from build123d import *

# Parameters (mm, degrees)
SKETCH1_R           = 1.73
BOSS_EXTRUDE1_DEPTH = 116
DOME1_FACE_RADIUS   = 1.73
DOME1_HEIGHT        = 5
DOME2_FACE_RADIUS   = 1.73
DOME2_HEIGHT        = 5


with BuildPart() as part:
    # Sketch1 → Boss-Extrude1 (new body)
    with BuildSketch(Plane.XY):
        with Locations(Location((0, 0, 0), (0, 0, 180))):
            Circle(SKETCH1_R)
    extrude(amount=BOSS_EXTRUDE1_DEPTH)

    # Dome1: a dome of height H over a round flat face of radius A is a cap of a sphere of radius (A * A + H * H) / (2 * H)
    dome1_r = (DOME1_FACE_RADIUS * DOME1_FACE_RADIUS + DOME1_HEIGHT * DOME1_HEIGHT) / (2 * DOME1_HEIGHT)
    dome1_base = Plane((0, 0, 0), z_dir=(0, 0, -1))
    with Locations(dome1_base.offset(DOME1_HEIGHT - dome1_r)):
        dome1_ball = Sphere(dome1_r, mode=Mode.PRIVATE)
    add(split(dome1_ball, bisect_by=dome1_base, keep=Keep.TOP, mode=Mode.PRIVATE))

    # Dome2: a dome of height H over a round flat face of radius A is a cap of a sphere of radius (A * A + H * H) / (2 * H)
    dome2_r = (DOME2_FACE_RADIUS * DOME2_FACE_RADIUS + DOME2_HEIGHT * DOME2_HEIGHT) / (2 * DOME2_HEIGHT)
    dome2_base = Plane((0, 0, 116), z_dir=(0, 0, 1))
    with Locations(dome2_base.offset(DOME2_HEIGHT - dome2_r)):
        dome2_ball = Sphere(dome2_r, mode=Mode.PRIVATE)
    add(split(dome2_ball, bisect_by=dome2_base, keep=Keep.TOP, mode=Mode.PRIVATE))


solid = part.part
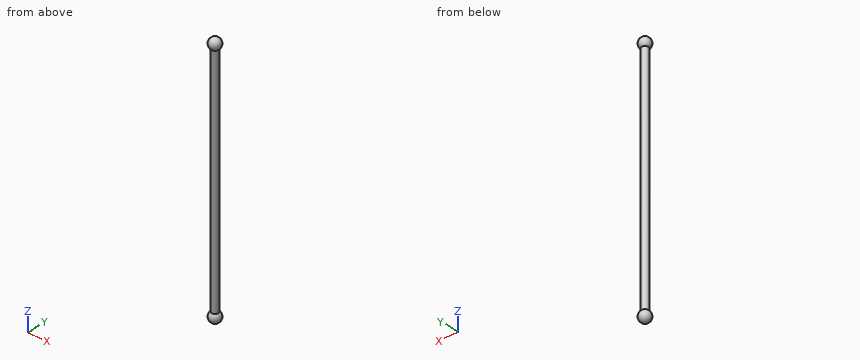
Input: part model. Units: mm. Frame: model coordinates. Round coordinates to 2 decimals unless told otherwise and drop trailing zeros. Loops run counter-clockwise (first coordinate to the right, second up) from the corner with the lowest first, then second, coordinate; pieces in that order, holes last. Notation, with made-up numbers: M 75.5,-23 L 83.5,-23 A9 cw 83.5,-7 Z; hole C 16,43 d8. An arc over 180 degrees is marked long. Answer as CSV lines item,"result". Start each with the question number.
(1) First-contact query: pin 1 (1.5 mm diameter, centred on x = 0, z = 54.5, fed in from +Y); pin 2 (1 mm diameter, centred on x = 0.5, y = 2, fed in from +Z). Flat tips, straight axial feed; report the tip coordinate or a pass-through.
(2) Section B-B, the plane z = 65. Output: boundary loops of the cut face in (x, y).
(3) Section A-A, the plane y = 0. Output: boundary loops of the cut face in (x, z).
(4) Line query: line 1 (Z direction, x = 2.1, y = 1.1); line 2 (Z direction, x = -2.5, y = 0.3); line 3 (Y direction, x = -0.7, z = 78). Output: solid intervals per line, ascending. Write a range as [from, to].
Values found:
1,pin 1,"stops at y = 1.73"
1,pin 2,"stops at z = 120.52"
2,outline,"C 0,0 d3.46"
3,outline,"M -1.73,0 A2.8 ccw long 1.73,0 L 1.73,116 A2.8 ccw long -1.73,116 Z"
4,line 1,"z = [-3.69, -0.71], [116.71, 119.69]"
4,line 2,"z = [-3.42, -0.98], [116.98, 119.42]"
4,line 3,"y = [-1.58, 1.58]"
